Could you check a few things on this model? Use its own coordinates, in mm. Give positions to 0.01 mm unless a question says otherwise; leave off trailing zeros. Loops run counter-clockwise (first coordinate to the right, second up) from the corner with the lowest first, then second, coordinate; pieces in that order, holes last. Notation, with made-up numbers: (81.25, 27.25) - (118.25, 27.25) arc R17 cw to (118.25, 39.25) - close; hole circle Ø4 at (74.25, 57). An arc over 180 degrees is marked (long way). One line per item, written item: value. Start each with the question number.
Q1. I want a section at B-B (z = -20). Please give me the cut outline in (x, y) (1 decimal), then the cut area to 3 significant figures.
Q2. I'm going to push flat-ended pins straight in: P1, Ø3, axis at x = -2.5, z = -8, coming from the -Y side; P2, Ø1.9, axis at y = 0, z = 66.04, coming from the -X side. Where does each tip first touch, or does it pass through?
Q3. If we mould it in two halves opening along Y, with no side actions, what happens to faces 1 (the face through (0, 0, -76.2)), 2 (the face through (-4.543, -1.431, 1.058)), 3 (the face through (-0.067, -0.608, 67.506))? For each: released by +Y, released by -Y, zero draft, split by the parting line, or undercut.
Q4. I want a section at A-A (z = 66.04). Please give me the cut outline in (x, y) (1 decimal).
Q5. If I drill on line 1 (Z direction, x = -2.75, y = -0.25); line 2 (Y direction, x = 0.5, z = 66.04); line 3 (Y direction, x = 0, z = 66.04), over which ranges is the centre line in solid material (lowest first)? Write a range as from..to.
```python
from build123d import *

# Parameters (mm, degrees)
SKETCH3_R           = 4.7625
BOSS_EXTRUDE1_DEPTH = 76.2
CHAMFER1_SIZE       = 0.47625
FILLET2_R           = 0.3571875
SKETCH4_R           = 1.5875
CUT_EXTRUDE1_DEPTH  = 362.708529549


with BuildPart() as part:
    # Sketch3 → Boss-Extrude1 (new, symmetric)
    with BuildSketch(Plane.XY):
        with Locations(Location((0, 0, 0), (0, 0, 180))):
            Circle(SKETCH3_R)
    extrude(amount=BOSS_EXTRUDE1_DEPTH, both=True)

    # Chamfer1
    chamfer1_edges = [part.edges().sort_by_distance(p)[0] for p in [
        (4.7625, 0, -76.2),
        (4.7625, 0, 76.2),
    ]]
    chamfer(chamfer1_edges, length=CHAMFER1_SIZE)

    # Fillet2
    fillet2_edges = [part.edges().sort_by_distance(p)[0] for p in [
        (4.7625, 0, -75.72375),
        (4.7625, 0, 75.72375),
    ]]
    fillet(fillet2_edges, radius=FILLET2_R)

    # Sketch4 → Cut-Extrude1 (cut, through all)
    with BuildSketch(Plane(origin=(-4.7625, -167.656009053, -241.627303232), x_dir=(0, 0, 1), z_dir=(-1, 0, 0))):
        with Locations((307.667303232, 167.656009053)):
            Circle(SKETCH4_R)
    extrude(amount=-CUT_EXTRUDE1_DEPTH, mode=Mode.SUBTRACT)


solid = part.part
```
Worked answers:
1. outline: circle Ø9.5 at (0, 0)
1. area: 71.3 mm²
2. P1: stops at y = -4.66
2. P2: passes through
3. face 1: zero draft
3. face 2: split by the parting line
3. face 3: undercut
4. outline: (-4.5, -1.6) arc R4.8 ccw to (4.5, -1.6) - close; (-4.5, 1.6) - (4.5, 1.6) arc R4.8 ccw to start
5. line 1: z = -76.2..64.47, 67.61..76.2
5. line 2: y = -4.74..-1.59, 1.59..4.74
5. line 3: y = -4.76..-1.59, 1.59..4.76
